from build123d import *

# Parameters (mm, degrees)
F1_DEPTH       = 23
F4_D           = 9
F4_DEPTH       = 15
F4_TIP         = 2.7038727856
F5_D           = 5
F5_DEPTH       = 15
F5_CBORE_D     = 9
F5_CBORE_DEPTH = 5
F5_TIP         = 1.5021515476
F6_R           = 5
F7_R           = 5
F8_R           = 1
F9_R           = 1


with BuildPart() as f1:
    # F0 (on Top) → F1 (new body, symmetric)
    with BuildSketch(Plane.XY):
        with BuildLine():
            Line((-13, 10), (-13, 0))
            ThreePointArc((-13, 0), (0, 13), (13, 0))
            Line((13, 0), (13, 10))
            Line((13, 10), (25.6173769149, 10))
            ThreePointArc((25.6173769149, 10), (0, 27.5), (-25.6173769149, 10))
            Line((-25.6173769149, 10), (-13, 10))
        make_face()
        with BuildLine():
            Line((-27.5, 0), (-13, 0))
            Line((-13, 0), (-13, 10))
            Line((-13, 10), (-25.6173769149, 10))
            ThreePointArc((-25.6173769149, 10), (-27.0252462076, 5.0878352391), (-27.5, 0))
        make_face()
        with BuildLine():
            Line((13, 10), (13, 0))
            Line((13, 0), (27.5, 0))
            ThreePointArc((27.5, 0), (27.0252462076, 5.0878352391), (25.6173769149, 10))
            Line((25.6173769149, 10), (13, 10))
        make_face()
        with BuildLine():
            Line((-27.5, 10), (-27.5, 0))
            ThreePointArc((-27.5, 0), (-27.0252462076, 5.0878352391), (-25.6173769149, 10))
            Line((-25.6173769149, 10), (-27.5, 10))
        make_face()
        with BuildLine():
            ThreePointArc((25.6173769149, 10), (27.0252462076, 5.0878352391), (27.5, 0))
            Line((27.5, 0), (27.5, 10))
            Line((27.5, 10), (25.6173769149, 10))
        make_face()
    extrude(amount=F1_DEPTH, both=True)

    # F4 (one way)
    with BuildSketch(Plane.XZ.offset(-10)):
        with Locations((20.25, 0), (-20.25, 0)):
            Circle(F4_D / 2)
    extrude(amount=-F4_DEPTH, mode=Mode.SUBTRACT)
    with Locations(Plane.XZ.offset(-10)):
        with Locations((20.25, 0), (-20.25, 0)):
            with Locations((0, 0, -(F4_DEPTH + F4_TIP / 2))):  # 118° drill point
                Cone(0, F4_D / 2, F4_TIP, mode=Mode.SUBTRACT)

    # F5
    with Locations(Plane(origin=(0, 10, 0), x_dir=(1, 0, 0), z_dir=(0, 1, 0))):
        with Locations((-20.25, 0), (20.25, 0)):
            CounterBoreHole(F5_D / 2, F5_CBORE_D / 2, F5_CBORE_DEPTH, depth=F5_DEPTH)
            with Locations((0, 0, -(F5_DEPTH + F5_TIP / 2))):  # 118° drill point
                Cone(0, F5_D / 2, F5_TIP, mode=Mode.SUBTRACT)

    # F6
    f6_edges = [f1.edges().sort_by_distance(p)[0] for p in [
        (27.5, 5, -23),
        (-27.5, 5, -23),
        (-26.558688, 10, -23),
        (0, 27.5, -23),
        (26.558688, 10, -23),
    ]]
    fillet(f6_edges, radius=F6_R)

    # F7
    f7_edges = [f1.edges().sort_by_distance(p)[0] for p in [
        (0, 27.5, 23),
        (26.558688, 10, 23),
        (-26.558688, 10, 23),
        (-27.5, 5, 23),
        (27.5, 5, 23),
    ]]
    fillet(f7_edges, radius=F7_R)

    # F8
    f8_edges = [f1.edges().sort_by_distance(p)[0] for p in [
        (27.5, 10, 0),
    ]]
    fillet(f8_edges, radius=F8_R)

    # F9
    f9_edges = [f1.edges().sort_by_distance(p)[0] for p in [
        (-27.5, 10, 0),
    ]]
    fillet(f9_edges, radius=F9_R)


solid = f1.part
The listing builds one solid part. Answer for the finished solid, in the listing's coordinates (mm). A direction names the side the tool comes from. Give positions to 0.01 mm unless a question says otherwise; leave off trailing zeros. Order: outer loops, then holes, each group sorted by start corner. A loop starts at its lowest first (then second) coordinate and runs counter-clockwise, first axis right, second up. Notation, with made-up numbers: (25, -14.5) - (54, -14.5) arc R17 cw to (54, 8.5) - close; hole circle Ø11 at (-19, 31.25). An arc over 180 degrees is marked (long way). Answer as CSV lines item,"result".
Q1. A cutting plane is placed at B-B, the plane y = 3.5. Determine the outline of the cut face in (x, z).
Answer key:
outline,"(-27.5, -18) arc R5 ccw to (-22.5, -23) - (-12.52, -23) - (-12.52, 23) - (-22.5, 23) arc R5 ccw to (-27.5, 18) - close; (12.52, -23) - (22.5, -23) arc R5 ccw to (27.5, -18) - (27.5, 18) arc R5 ccw to (22.5, 23) - (12.52, 23) - close; hole circle Ø5 at (-20.25, 0); hole circle Ø5 at (20.25, 0)"
Q2. Determine the mould class of faces 1 (the face through (-17, 0, 0)), 2 (the face through (0, 14, -23)), 3 (the face through (-17.752, 2.465, -0.11)) for opening direction Z: pulls with the +Z half, pulls with the -Z half, needs draft (parallel to the pull), parting line crosses it, or undercut.
Answer key:
face 1,"needs draft"
face 2,"pulls with the -Z half"
face 3,"undercut"
Q3. Which of the six approach directions +Z, -Z, +X, -X, +Y, -Y give full straight-line access (tool end or side, diameter ignored) to faces 4 (the face through (25.05, 8.75, -21.31)), 5 (the face through (25.05, 8.72, 21.34)), 6 (the face through (-18, 5, 2))?
Answer key:
face 4,"-Z, +X, +Y"
face 5,"+Z, +X, +Y"
face 6,"+Y"
Q4. Straight lines are drawn through the part: L1, parallel to Z at x = -20.25, y = 4.05; L2, parallel to X at y = 16, z = 0; L3, parallel to Y at x = -21, z = 9.5. For each, find the intervals that lie inside material, in ascending order.
Answer key:
L1,"z = -23 to -2.5, 2.5 to 23"
L2,"x = -15.75 to 15.75"
L3,"y = 0 to 17.76"
Q5. A cutting plane is placed at C-C, the plane x = 0. Determine the outline of the cut face in (y, z), and give its area (3 significant figures).
Answer key:
outline,"(13, -23) - (22.5, -23) arc R5 ccw to (27.5, -18) - (27.5, 18) arc R5 ccw to (22.5, 23) - (13, 23) - close"
area,"656 mm^2"
Q6. Each of these flat-tipped pins is pushed along its axis until it touches: pin 1 Ø10 at (x, z) = (-22.5, 2) entering from +Y; pin 2 Ø2.5 at (x, z) = (19.5, -2) entering from +Y; pin 3 Ø10.5 at (x, z) = (-20.25, 0) entering from +Y. Where does it stop, or does it pass through?
Answer key:
pin 1,"stops at y = 20.93"
pin 2,"stops at y = 5"
pin 3,"stops at y = 23.05"
Q7. A cutting plane is placed at A-A, the plane z = 0. Determine the outline of the cut face in (x, y).
Answer key:
outline,"(-27.5, 0) - (-22.75, 0) - (-22.75, 5) - (-24.75, 5) - (-24.75, 11.99) arc R27.5 ccw to (-25.62, 10) - (-26.5, 10) arc R1 ccw to (-27.5, 9) - close; (-17.75, 0) - (-13, 0) arc R13 cw to (13, 0) - (17.75, 0) - (17.75, 5) - (15.75, 5) - (15.75, 22.54) arc R27.5 ccw to (-15.75, 22.54) - (-15.75, 5) - (-17.75, 5) - close; (22.75, 0) - (27.5, 0) - (27.5, 9) arc R1 ccw to (26.5, 10) - (25.62, 10) arc R27.5 ccw to (24.75, 11.99) - (24.75, 5) - (22.75, 5) - close"
Q8. A cutting plane is placed at D-D, the plane z = 13.5. Determine the outline of the cut face in (x, y).
Answer key:
outline,"(-27.5, 0) - (-13, 0) arc R13 cw to (13, 0) - (27.5, 0) - (27.5, 9) arc R1 ccw to (26.5, 10) - (25.62, 10) arc R27.5 ccw to (-25.62, 10) - (-26.5, 10) arc R1 ccw to (-27.5, 9) - close"
